Here's how the part is built. I have some questions about the finished solid (model axes, mm). A direction names the side the tool comes from. Give positions to 0.01 mm unless a question says otherwise; leave off trailing zeros. Write each loop counter-clockwise with the first axis right and the second up, starting at its lowest first coordinate (ties: lowest second). Pieces come first, ordered by that corner, then holes. Notation, with made-up numbers: (68, 9) - (97, 9) arc R34 cw to (97, 44) - close; hole circle Ø9 at (4, 31.5). An arc over 180 degrees is marked (long way). Use a Markdown table: item, result.
Autodesk Inventor part; units mm, degrees
ref_plane "YZ Plane" through (0, 0, 0) normal (1, 0, 0) x (0, 1, 0)
ref_plane "XZ Plane" through (0, 0, 0) normal (0, 1, 0) x (-1, 0, 0)
ref_plane "XY Plane" through (0, 0, 0) normal (0, 0, 1) x (1, 0, 0)
sketch "Sketch1" plane through (0, 0, 0) normal (0, 0, 1) x (1, 0, 0)
  line L0 (-23.5, 23.5) -> (-23.5, -23.5)
  line L1 (23.5, 23.5) -> (-23.5, 23.5)
  line L2 (23.5, -23.5) -> (23.5, 23.5)
  line L3 (-23.5, -23.5) -> (23.5, -23.5)
  circle A0 centre (-18, -18) radius 1.4
  circle A1 centre (-18, 18) radius 1.4
  circle A2 centre (18, 18) radius 1.4
  circle A3 centre (18, -18) radius 1.4
  line L4 (12.5, 12) -> (12.5, -12)
  line L5 (-12.5, -12) -> (-12.5, 12)
  line L6 (-12.5, 12) -> (12.5, 12)
  line L7 (12.5, -12) -> (12.5, -23.5)
  line L8 (-12.5, -12) -> (-12.5, -23.5)
  point P0 (0, 0)
extrude "Extrusion1" add sketch "Sketch1" along normal blind 3 contours L1 L2 L3 L7 L4 L6 L5 L8 L0
properties part number "Camera-Holder_Mount-Bottom"
Item 1: If we section it at B-B, the plane y = 18: Write out the boundary of the cut face in (x, z), plus the area to 3 significant figures.
Values:
| item | result |
|---|---|
| outline | (-23.5, 0) - (-19.4, 0) - (-19.4, 3) - (-23.5, 3) - close; (-16.6, 0) - (16.6, 0) - (16.6, 3) - (-16.6, 3) - close; (19.4, 0) - (23.5, 0) - (23.5, 3) - (19.4, 3) - close |
| area | 124 mm2 |
Item 2: Thinking about a two-plate mould opening in Y: for faces 3 (the flat face through (0, 23.5, 1)), 4 (the flat face through (-18, -23.5, 1)), 5 (the flat face through (0, 16, 0)), 6 (the cylindrical face through (-19.4, 17.94, 1.48)), which applies, +Y half, -Y half, draft (parallel to the pull), parting line (faces both ways), or undercut?
Values:
| item | result |
|---|---|
| face 3 | +Y half |
| face 4 | -Y half |
| face 5 | draft |
| face 6 | undercut |
Item 3: I need wall thicknesses on line 1 along X through (y, z) = (-8, 1.45); line 2 along Y through (x, z) = (-2.5, 2.45). Which ranges of each line are inside material? Lowest first, please. Write a range as [from, to].
Values:
| item | result |
|---|---|
| line 1 | x = [-23.5, -12.5], [12.5, 23.5] |
| line 2 | y = [12, 23.5] |
Item 4: If we section it at D-D, the plane z = 2.4: Write out the boundary of the cut face in (x, y).
Values:
| item | result |
|---|---|
| outline | (-23.5, -23.5) - (-12.5, -23.5) - (-12.5, 12) - (12.5, 12) - (12.5, -23.5) - (23.5, -23.5) - (23.5, 23.5) - (-23.5, 23.5) - close; hole circle Ø2.8 at (-18, -18); hole circle Ø2.8 at (-18, 18); hole circle Ø2.8 at (18, -18); hole circle Ø2.8 at (18, 18) |
Item 5: For faces 1 (the flat face through (0, 12, 1)), 2 (the flat face through (18, -23.5, 1)), which set-ups out of +Z, -Z, +X, -X, +Y, -Y let a thin tool reach every point of the face, with its end or its side?
Values:
| item | result |
|---|---|
| face 1 | +Z, -Z, -Y |
| face 2 | +Z, -Z, +X, -X, -Y |
Item 6: If we section it at A-A, the plane y = 5: Write out the boundary of the cut face in (x, z).
Values:
| item | result |
|---|---|
| outline | (-23.5, 0) - (-12.5, 0) - (-12.5, 3) - (-23.5, 3) - close; (12.5, 0) - (23.5, 0) - (23.5, 3) - (12.5, 3) - close |
